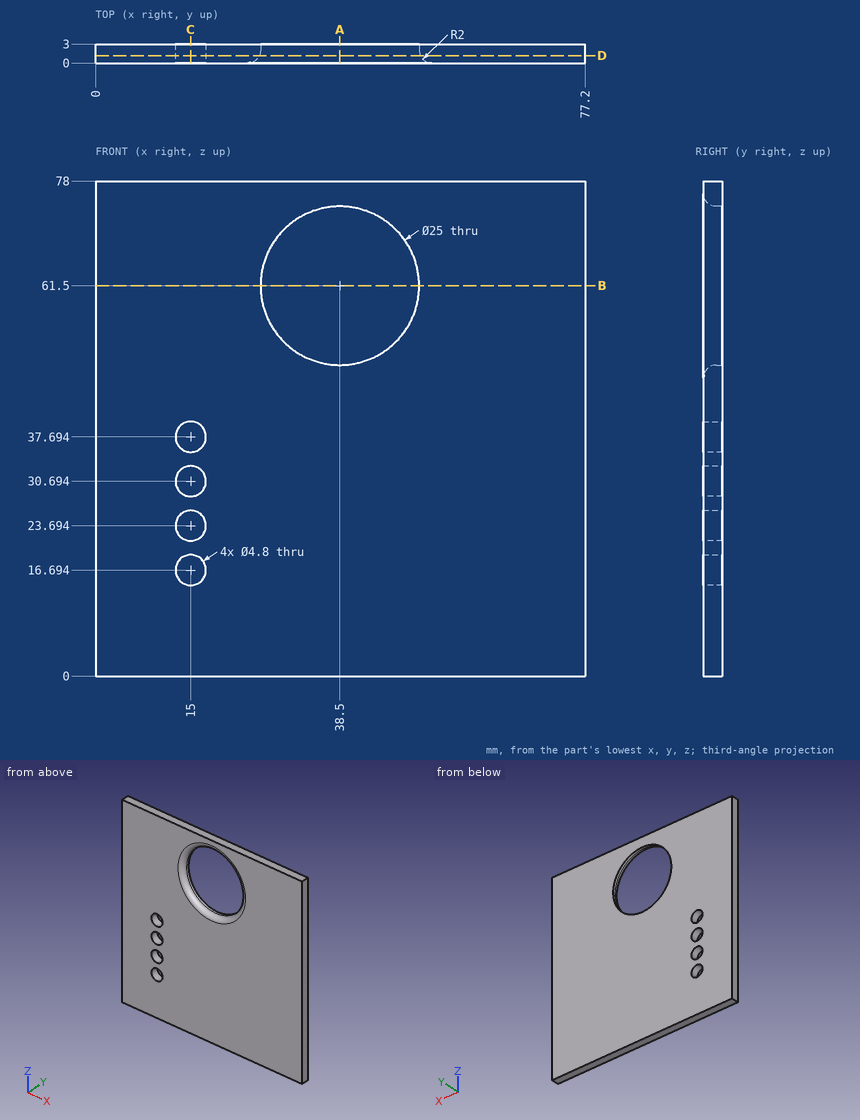
Design review of the part shown in the three views and the two pictorial views. Dimensions are in mm from the part's minimum x, y and z. Round coordinates to 2 decimals unless told otherwise and drop trailing zeros. Loops run counter-clockwise (first coordinate to the right, second up) from the corner with the lowest first, then second, coordinate; pieces in that order, holes last. Notation, with made-up numbers: M 59,84 L 102,84 A6 cw 102,91 Z; hole C 70.5,86.5 d9. An arc over 180 degrees is marked long. Write item = value, one per line.
Item 1: Take a section at A-A on x = 38.5. Write out the cut boundary in (y, z).
Return value:
outline = M 0,0 L 3,0 L 3,49 L 2,49 A2 ccw 0,47 Z; M 0,76 A2 ccw 2,74 L 3,74 L 3,78 L 0,78 Z
Item 2: Take a section at C-C on x = 15. Write out the cut boundary in (y, z).
Return value:
outline = M 0,0 L 3,0 L 3,14.29 L 0,14.29 Z; M 0,19.09 L 3,19.09 L 3,21.29 L 0,21.29 Z; M 0,26.09 L 3,26.09 L 3,28.29 L 0,28.29 Z; M 0,33.09 L 3,33.09 L 3,35.29 L 0,35.29 Z; M 0,40.09 L 3,40.09 L 3,78 L 0,78 Z
Item 3: Take a section at D-D on y = 1.15. Write out the cut boundary in (x, z).
Return value:
outline = M 0,0 L 77.2,0 L 77.2,78 L 0,78 Z; hole C 15,16.69 d4.8; hole C 15,23.69 d4.8; hole C 15,30.69 d4.8; hole C 15,37.69 d4.8; hole C 38.5,61.5 d25.38
Item 4: Take a section at B-B on z = 61.5. Write out the cut boundary in (x, y).
Return value:
outline = M 0,0 L 24,0 A2 ccw 26,2 L 26,3 L 0,3 Z; M 51,2 A2 ccw 53,0 L 77.2,0 L 77.2,3 L 51,3 Z
Item 5: Insertion check: P1, Ø3, axis at x = 48, z = 63.5, coming from the +Y side. The pin has a flat end and moves straight along its axis. Give the tip position at first contact, or say it passes through.
Return value:
P1 = through
Item 6: For line 1 (Z direction, x = 15, y = 2.35); line 2 (Z direction, x = 13, y = 1.2) (1 decimal); line 3 (X direction, y = 1.25, z = 56.5) (1 decimal), list the stretches that pass through material, from the lowest coordinate up. Write a range as [from, to].
Return value:
line_1 = [0, 14.29], [19.09, 21.29], [26.09, 28.29], [33.09, 35.29], [40.09, 78]
line_2 = [0, 15.4], [18, 22.4], [25, 29.4], [32, 36.4], [39, 78]
line_3 = [0, 26.9], [50.1, 77.2]
